```python
from build123d import *

# Parameters (mm, degrees)
SKETCH1_W           = 13.081
SKETCH1_H           = 17.907
BOSS_EXTRUDE1_DEPTH = 14.1859
SKETCH2_W           = 13.081
SKETCH2_H           = 3.2258
BOSS_EXTRUDE2_DEPTH = 11.9253
CHAMFER1_SIZE       = 2.54
FILLET1_R           = 2.54
SKETCH3_R           = 2.63525
CUT_EXTRUDE1_DEPTH  = 3.2258
SKETCH4_R           = 1.75
CUT_EXTRUDE2_DEPTH  = 29.367905597


with BuildPart() as part:
    # Sketch1 → Boss-Extrude1 (new body)
    with BuildSketch(Plane.XY):
        Rectangle(SKETCH1_W, SKETCH1_H)
    extrude(amount=BOSS_EXTRUDE1_DEPTH)

    # Sketch2 → Boss-Extrude2 (add)
    with BuildSketch(Plane.XY.offset(14.1859)):
        with Locations((0, -7.3406)):
            Rectangle(SKETCH2_W, SKETCH2_H)
    extrude(amount=BOSS_EXTRUDE2_DEPTH)

    # Chamfer1
    chamfer1_edges = [part.edges().sort_by_distance(p)[0] for p in [
        (0, 8.9535, 14.1859),
    ]]
    chamfer(chamfer1_edges, length=CHAMFER1_SIZE)

    # Fillet1
    fillet1_edges = [part.edges().sort_by_distance(p)[0] for p in [
        (-6.5405, -7.3406, 26.1112),
        (6.5405, -7.3406, 26.1112),
    ]]
    fillet(fillet1_edges, radius=FILLET1_R)

    # Sketch3 → Cut-Extrude1 (cut)
    with BuildSketch(Plane(origin=(0, -5.7277, 0), x_dir=(1, 0, 0), z_dir=(0, 1, 0))):
        with Locations(Location((0, -20.14855, 0), (0, 0, 270))):
            Circle(SKETCH3_R)
    extrude(amount=-CUT_EXTRUDE1_DEPTH, mode=Mode.SUBTRACT)

    # Sketch4 → Cut-Extrude2 (cut, through all)
    with BuildSketch(Plane(origin=(0, 0, 0), x_dir=(-1, 0, 0), z_dir=(0, 0, -1))):
        with Locations((0, 5.1334)):
            Circle(SKETCH4_R)
        with Locations((0, -3.4466)):
            Circle(SKETCH4_R)
    extrude(amount=-CUT_EXTRUDE2_DEPTH, mode=Mode.SUBTRACT)


solid = part.part
```
Could you check a few things on this model? Use its own coordinates, in mm. A direction names the side the tool comes from. Round coordinates to 2 decimals unless told otherwise and drop trailing zeros. Loops run counter-clockwise (first coordinate to the right, second up) from the corner with the lowest first, then second, coordinate; pieces in that order, holes last. Notation, with made-up numbers: (21, 59) -> (65, 59) arc R25 ccw to (65, 96) -> close; hole circle Ø5 at (16, -29). An arc over 180 degrees is marked (long way). One line per question, with ' | ' between items.
(1) If we section it at A-A on y = -7.5: List the corners of the cut face in (x, z) for me, and give its area (3 significant figures).
Model answer:
outline: (-6.54, 0) -> (6.54, 0) -> (6.54, 23.57) arc R2.54 ccw to (4, 26.11) -> (-4, 26.11) arc R2.54 ccw to (-6.54, 23.57) -> close; hole circle Ø5.27 at (0, 20.15) | area: 317 mm^2
(2) If I drill on probe 1 along Y at (x, z) = (0, 10.25); probe 2 along X at (y, z) = (5, 4); probe 3 along Z at (x, y) = (-0.5, 0.5), over which ranges is the centre line in solid material (lowest first)?
Model answer:
probe 1: y = -8.95 to -5.2, -1.7 to 3.38, 6.88 to 8.95 | probe 2: x = -6.54 to -1.74, 1.74 to 6.54 | probe 3: z = 0 to 14.19
(3) For pin 1 Ø2 at (x, z) = (-2.5, 14) entering from +Y; pin 2 Ø3.5 at (x, y) = (1, -0.5) entering from +Z, each with a flat end and sliding along its axis, tell me the tip position at first contact or that it passes through.
Model answer:
pin 1: stops at y = 7.6 | pin 2: stops at z = 14.19
(4) Thinking about a two-plate mould opening in X: for faces 3 (the face through (0.116, -7.318, 17.516)), 4 (the face through (-6.54, -2, 9)), 5 (the face through (0, 0, 0)), which applies, released by +X, released by -X, zero draft, split by the parting line, or undercut?
Model answer:
face 3: undercut | face 4: released by -X | face 5: zero draft
(5) If we section it at D-D on y = -2: List the corners of the cut face in (x, z) for me.
Model answer:
outline: (-6.54, 0) -> (-0.98, 0) -> (-0.98, 14.19) -> (-6.54, 14.19) -> close; (0.98, 0) -> (6.54, 0) -> (6.54, 14.19) -> (0.98, 14.19) -> close
(6) If we section it at C-C on z = 21.75: List the corners of the cut face in (x, y) for me, and give its area (3 significant figures).
Model answer:
outline: (-6.54, -8.95) -> (-2.09, -8.95) -> (-2.09, -5.73) -> (-6.54, -5.73) -> close; (2.09, -8.95) -> (6.54, -8.95) -> (6.54, -5.73) -> (2.09, -5.73) -> close | area: 28.7 mm^2
(7) If we section it at B-B on x = 0: List the corners of the cut face in (y, z) for me.
Model answer:
outline: (-8.95, 0) -> (-5.2, 0) -> (-5.2, 14.19) -> (-5.73, 14.19) -> (-5.73, 17.51) -> (-8.95, 17.51) -> close; (-8.95, 22.78) -> (-5.73, 22.78) -> (-5.73, 26.11) -> (-8.95, 26.11) -> close; (-1.7, 0) -> (3.38, 0) -> (3.38, 14.19) -> (-1.7, 14.19) -> close; (6.88, 0) -> (8.95, 0) -> (8.95, 11.65) -> (6.88, 13.72) -> close
(8) For faces 1 (the face through (0, 0, 14.186)), 2 (the face through (0, -7, 26.111)), which set-ups out of +Z, -Z, +X, -X, +Y, -Y let a thin tool reach every point of the face, with its end or its side?
Model answer:
face 1: +Z, +X, -X, +Y | face 2: +Z, +X, -X, +Y, -Y
